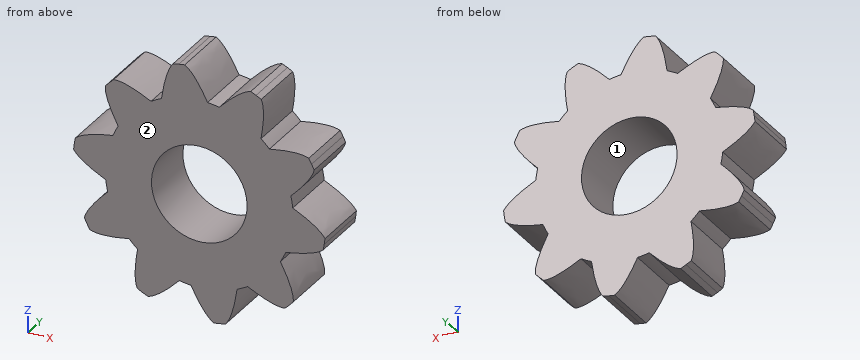
from build123d import *

# Parameters (mm, degrees)
SKETCH1_R           = 7.957747155
BOSS_EXTRUDE4_DEPTH = 5
CIRPATTERN6_COUNT   = 10
SKETCH2_R           = 4.05
CUT_EXTRUDE1_DEPTH  = 10


with BuildPart() as part:
    # Sketch1 → Boss-Extrude4 (new body)
    with BuildSketch(Plane(origin=(0, 0, 0), x_dir=(1, 0, 0), z_dir=(0, 1, 0))):
        Circle(SKETCH1_R)
        with BuildLine():
            ThreePointArc((7.958110252, 7.164089255), (7.788629845, 7.347988758), (7.614900879, 7.527880064))
            ThreePointArc((7.614900879, 7.527880064), (7.43701812, 7.703665045), (7.255078601, 7.875247815))
            add(Edge.make_bspline(
                [(7.255078601, 7.875247815), (6.306550312, 7.97741942), (4.090117658, 6.826175893)],
                knots=[0.62632571, 0.62632571, 0.62632571, 1, 1, 1], degree=2))
            ThreePointArc((4.090117658, 6.826175893), (5.659220003, 5.594548126), (6.872732742, 4.011394325))
            add(Edge.make_bspline(
                [(6.872732742, 4.011394325), (8.04937368, 6.214449356), (7.958110252, 7.164089255)],
                knots=[0, 0, 0, 0.37367429, 0.37367429, 0.37367429], degree=2))
        make_face()
    boss_extrude4 = extrude(amount=BOSS_EXTRUDE4_DEPTH)

    # CirPattern6: Boss-Extrude4 ×10 about axis
    cirpattern6_axis = Axis((0, 0, 0), (0, -1, 0))
    for i in range(1, CIRPATTERN6_COUNT):
        add(boss_extrude4.rotate(cirpattern6_axis, i * 360 / CIRPATTERN6_COUNT))

    # Sketch2 → Cut-Extrude1 (cut)
    with BuildSketch(Plane(origin=(0, 5, 0), x_dir=(1, 0, 0), z_dir=(0, 1, 0))):
        with Locations(Location((0, 0, 0), (0, 0, 270))):
            Circle(SKETCH2_R)
    extrude(amount=-CUT_EXTRUDE1_DEPTH, mode=Mode.SUBTRACT)


solid = part.part
Geometry: final body of the model. Coordinates: model frame, mm. Face numbers are marked on the shaded views. Round coordinates to 2 decimals unless told otherwise and drop trailing zeros.
Q1. Pin query (flat end, axial travel): pin 1 (1.5 mm diameter, centred on y = 2, z = 0.5, fed in from +X); pin 2 (3 mm diameter, centred on y = 4, z = 3.5, fed in from +X); pin 3 (1 mm diameter, centred on x = 6.5, y = 2, fed in from -Z); pin 4 (6.5 mm diameter, centred on x = 0, z = 0, fed in from +Y). Return the tip coordinate at first contact, or that it passes through.
Result sheet:
pin 1: stops at x = 9.75
pin 2: stops at x = 9.73
pin 3: stops at z = -7.88
pin 4: passes through
Q2. Material intervals for probe 1 along Z at (x, y) = (0.25, 4.8); probe 2 along X at (y, z) = (4, -2.5); probe 3 along X at (y, z) = (4.35, 1.75), sorted ascending.
Result sheet:
probe 1: z = -9.59 to -4.04, 4.04 to 8.78
probe 2: x = -8.45 to -3.19, 3.19 to 9.84
probe 3: x = -10.56 to -3.65, 3.65 to 7.76
Q3. Mould query, pull axis Z, two halves, no side actions, for the marked faces 1 and 2. Classes: released by +Z, released by -Z, zero draft, split by the parting line, or undercut.
Result sheet:
face 1: undercut
face 2: zero draft
